Print and shaded views of the part. All mm, measured from the part's lowest x, y and z. Round coordinates to 2 decimals unless told otherwise and drop trailing zeros. Loops run counter-clockwise (first coordinate to the right, second up) from the corner with the lowest first, then second, coordinate; pieces in that order, holes last. Notation, with made-up numbers: (-10, -34.5) - (35, -34.5) arc R24 ccw to (35, 0.5) - close; hole circle Ø10 at (-21, 54.5). An arc over 180 degrees is marked (long way). Use one line per item in the form item = value.
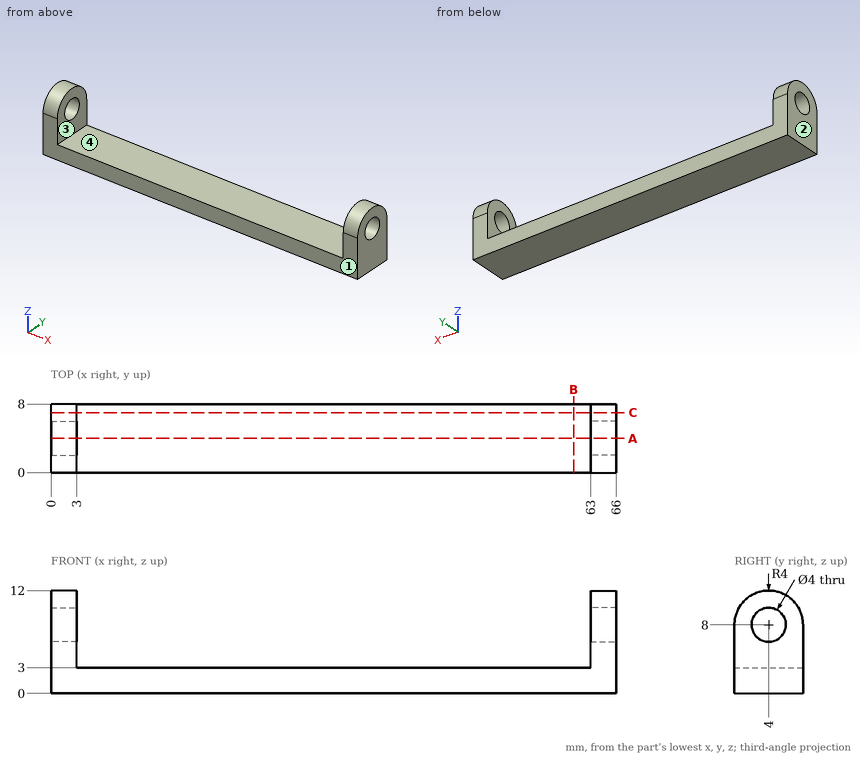
1. Cut at B-B, the plane x = 61. Give the cut face in (y, z), plus the area to 3 significant figures.
Geometry check:
outline = (0, 0) - (8, 0) - (8, 3) - (0, 3) - close
area = 24.0 mm^2
2. Cut at C-C, the plane y = 7. Give the cut face in (x, z), plus the area to 3 significant figures.
Geometry check:
outline = (0, 0) - (66, 0) - (66, 10.65) - (63, 10.65) - (63, 3) - (3, 3) - (3, 10.65) - (0, 10.65) - close
area = 244 mm^2
3. Flat gauge pins, fed straight in: pin 1 (2.5 mm diameter, centred on y = 5.5, z = 7, fed in from +X); pin 2 (3.5 mm diameter, centred on y = 4, z = 8, fed in from -X); pin 3 (4 mm diameter, centred on x = 20.5, y = 4.5, fed in from +Z). Where does each tip first touch, or does it go through?
Geometry check:
pin_1 = 66
pin_2 = through
pin_3 = 3
4. Wall check: probe 1 along Z at (x, y) = (63.7, 4); probe 2 along X at (y, z) = (2, 5); probe 3 along Y at (x, z) = (64.9, 8). Give the ranges that are in metal, low to high.
Geometry check:
probe_1 = 0 to 6, 10 to 12
probe_2 = 0 to 3, 63 to 66
probe_3 = 0 to 2, 6 to 8
5. Pull direction X, two halves, no side cores. Call the marked faces 1, 2, 3 and 4: +X half, -X half, draft (parallel to the pull), parting line (faces both ways), or undercut.
Geometry check:
face_1 = draft
face_2 = -X half
face_3 = undercut
face_4 = undercut
6. Cut at A-A, the plane y = 4. Give the cut face in (x, z).
Geometry check:
outline = (0, 0) - (66, 0) - (66, 6) - (63, 6) - (63, 3) - (3, 3) - (3, 6) - (0, 6) - close; (0, 10) - (3, 10) - (3, 12) - (0, 12) - close; (63, 10) - (66, 10) - (66, 12) - (63, 12) - close
